Drawing for the job (mm, zero at the part's lowest x, y, z). A direction names the side the tool comes from. Coordinates: 2 decimals unless noted, no trailing zeros. Write each loop counter-clockwise with the first axis right and the second up, starting at its lowest first coordinate (ties: lowest second). Pieces come first, ordered by that corner, then holes. Notation, with made-up numbers: M 37,73 L 57,73 A18 ccw 57,95 Z; hole C 20.5,42 d3. An arc over 180 degrees is marked long. Use a Markdown table: item, result. Add a question column.
Q1. Slice it at B-B on x = 12.5. Write the cut outline in (y, z).
Q2. Wall check: L1, parallel to Z at x = 2.3, y = 55; L2, parallel to Y at x = 22.5, z = 35.5. Give the ranges that are in metal, low to high. Write a range as from..to.
Q3. Pin check, flat tips, straight feed: pin 1 Ø1.8 at (x, y) = (2, 26) entering from -Z; pin 2 Ø0.9 at (x, y) = (1, 53.5) entering from -Z; pin 3 Ø2.5 at (y, z) = (1, 9.5) entering from -X; pin 4 Ø3.5 at (y, z) = (55, 37.5) entering from -X. Stop position of each tip, or through.
Q4. Slice it at A-A on z = 22.5. Write the cut outline in (x, y), then the cut area to 3 significant figures.
Q5. Tool access for the marked faces 1 and 2: list every direction of +Z, -Z, +X, -X, +Y, -Y with a clear straight run to the whole face (end or side of a thin tool).
Q6. Slice it at C-C on y = 15. Write the cut outline in (x, z).
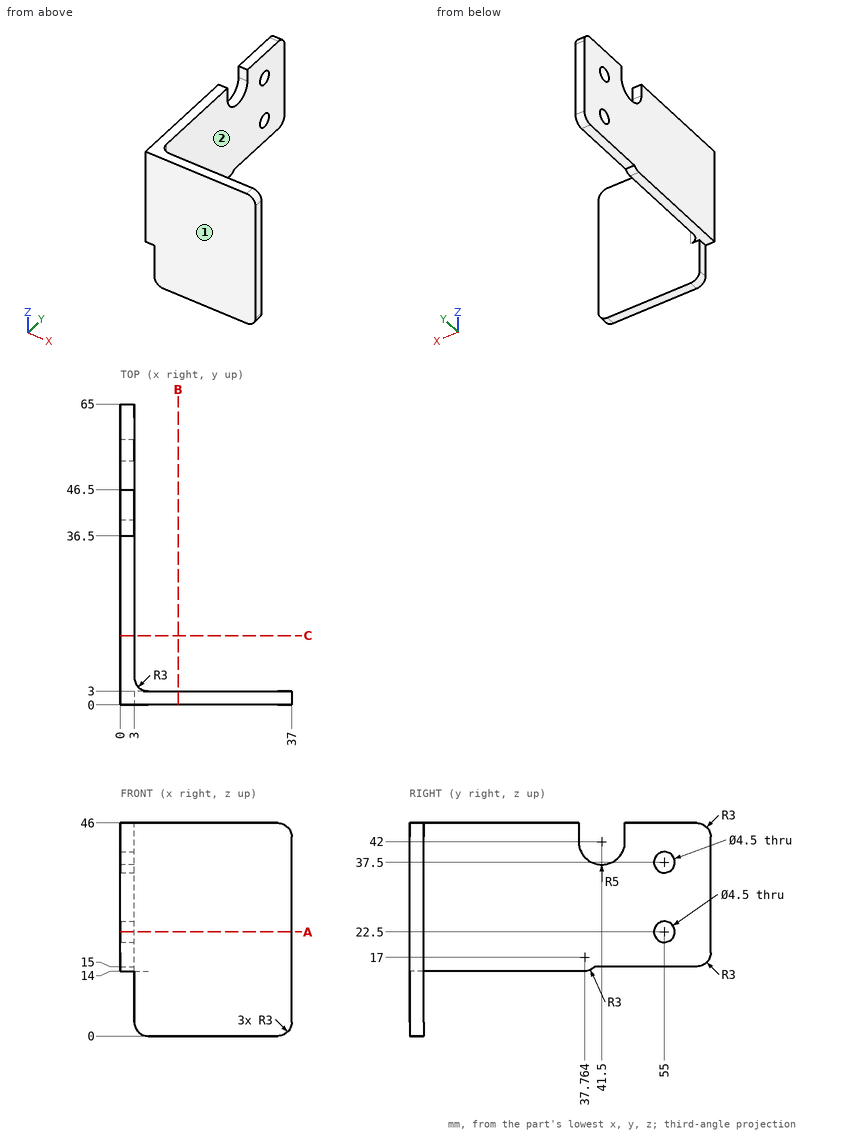
Recorded:
| question | item | result |
|---|---|---|
| 1 | outline | M 0,0 L 3,0 L 3,46 L 0,46 Z |
| 2 | L1 | 15..20.25, 24.75..35.25, 39.75..46 |
| 2 | L2 | 0..3 |
| 3 | pin 1 | z = 14 |
| 3 | pin 2 | z = 15 |
| 3 | pin 3 | x = 3 |
| 3 | pin 4 | through |
| 4 | outline | M 0,0 L 37,0 L 37,3 L 6,3 A3 cw 3,6 L 3,52.75 L 0,52.75 Z; M 0,57.25 L 3,57.25 L 3,65 L 0,65 Z |
| 4 | area | 285 mm² |
| 5 | face 1 | +Z, -Z, +X, -X, -Y |
| 5 | face 2 | +Z, -Z, +X, +Y |
| 6 | outline | M 0,14 L 3,14 L 3,46 L 0,46 Z |
